Here's how the part is built. I have some questions about the finished solid (model axes, mm). Coordinates: 2 decimals unless noted, no trailing zeros. Write each loop counter-clockwise with the first axis right and the second up, starting at its lowest first coordinate (ties: lowest second). Pieces come first, ordered by that corner, then holes. Notation, with made-up numbers: (-5, 58.5) - (19, 58.5) arc R13 cw to (19, 62.5) - close; hole circle Ø3 at (-39.5, 62.5). An arc over 180 degrees is marked (long way). Answer in a Markdown table with one row per item. Add a question column.
Item 1: Imagine slicing it at B-B (y = 12.5). Please give me the cut outline in (x, z), plus the area to 3 significant figures.
Item 2: If I drill on probe 1 along X at (y, z) = (10.5, 3.5); probe 2 along X at (y, z) = (-13, 27.5); probe 3 along Z at (x, y) = (53, 25.5), over which ranges is the centre line in solid material (lowest first)? Write a range as from..to.
Item 3: We'd pull the mould along Z, two halves only. Please class faces 1 (the face through (136, 0, 33.33)), 2 (the face through (136, 0, -27.863)), 3 (the face through (-106.496, 0.444, 10.456)): +Z half, -Z half, draft (parallel to the pull), parting line (faces both ways), or undercut.
Item 4: Imagine slicing it at A-A (z = 8). Please give me the cut outline in (x, y).
from build123d import *

# Parameters (mm, degrees)
F0_W     = 508
F0_H     = 61.19313
F0_R     = 5.334
F0_R_2   = 11.43
F0_R_3   = 5.338674
F1_DEPTH = 31.75


with BuildPart() as f1:
    # F0 (on Front) → F1 (new body, symmetric)
    with BuildSketch(Plane.XZ):
        with Locations((139.418788, 2.733509)):
            Rectangle(F0_W, F0_H)
        with Locations((55.385654, -19.760456)):
            Circle(F0_R, mode=Mode.SUBTRACT)
        with Locations((-98.071212, 2.731244)):
            Circle(F0_R_2, mode=Mode.SUBTRACT)
        with Locations((175.385654, -19.760456)):
            Circle(F0_R, mode=Mode.SUBTRACT)
        with Locations((55.385654, 25.239544)):
            Circle(F0_R_3, mode=Mode.SUBTRACT)
        with Locations((175.385654, 25.239544)):
            Circle(F0_R, mode=Mode.SUBTRACT)
    extrude(amount=F1_DEPTH, both=True)


solid = f1.part
Here are the results:
| question | item | result |
|---|---|---|
| 1 | outline | (-114.58, -27.86) - (393.42, -27.86) - (393.42, 33.33) - (-114.58, 33.33) - close; hole circle Ø22.86 at (-98.07, 2.73); hole circle Ø10.67 at (55.39, -19.76); hole circle Ø10.68 at (55.39, 25.24); hole circle Ø10.67 at (175.39, -19.76); hole circle Ø10.67 at (175.39, 25.24) |
| 1 | area | 30,300 mm2 |
| 2 | probe 1 | x = -114.58..-109.48, -86.67..393.42 |
| 2 | probe 2 | x = -114.58..50.55, 60.22..170.55, 180.22..393.42 |
| 2 | probe 3 | z = -27.86..-24.53, -14.99..20.46, 30.02..33.33 |
| 3 | face 1 | +Z half |
| 3 | face 2 | -Z half |
| 3 | face 3 | undercut |
| 4 | outline | (-114.58, -31.75) - (-108.21, -31.75) - (-108.21, 31.75) - (-114.58, 31.75) - close; (-87.93, -31.75) - (393.42, -31.75) - (393.42, 31.75) - (-87.93, 31.75) - close |
